from build123d import *

# Parameters (mm, degrees)
SKETCH1_R                = 55.5
BOSS_EXTRUDE1_DEPTH      = 7
CUT_EXTRUDE1_DEPTH       = 7
FILLET1_R                = 5
CIRPATTERN1_COUNT        = 7
FILLET1_OF_CIRPATTERN1_R = 5
SKETCH3_R                = 5
BOSS_EXTRUDE2_DEPTH      = 4.1


with BuildPart() as part:
    # Sketch1 → Boss-Extrude1 (new body)
    with BuildSketch(Plane(origin=(0, 0, 0), x_dir=(1, 0, 0), z_dir=(0, 1, 0))):
        with Locations(Location((0, 0, 0), (0, 0, 270))):
            Circle(SKETCH1_R)
    extrude(amount=BOSS_EXTRUDE1_DEPTH)

    # Sketch2 → Cut-Extrude1 (cut)
    with BuildSketch(Plane(origin=(0, 7, 0), x_dir=(1, 0, 0), z_dir=(0, 1, 0))):
        with BuildLine():
            Line((0, 15), (0, 45.5))
            ThreePointArc((0, 45.5), (15.561916521, 42.756014246), (29.246836241, 34.855022162))
            Line((29.246836241, 34.855022162), (9.641814145, 11.490666647))
            ThreePointArc((9.641814145, 11.490666647), (5.13030215, 14.095389312), (0, 15))
        make_face()
    cut_extrude1 = extrude(amount=-CUT_EXTRUDE1_DEPTH, mode=Mode.SUBTRACT)

    # Fillet1
    fillet1_edges = [part.edges().sort_by_distance(p)[0] for p in [
        (9.641814145, 3.5, -11.490666647),
        (0, 3.5, -15),
        (0, 3.5, -45.5),
        (29.246836241, 3.5, -34.855022162),
    ]]
    fillet(fillet1_edges, radius=FILLET1_R)

    # CirPattern1: Cut-Extrude1 ×7 about axis
    cirpattern1_axis = Axis((0, 0, 0), (0, 1, 0))
    for i in range(1, CIRPATTERN1_COUNT):
        add(cut_extrude1.rotate(cirpattern1_axis, i * 360 / CIRPATTERN1_COUNT), mode=Mode.SUBTRACT)

    # Fillet1 of CirPattern1
    fillet1_of_cirpattern1_edges = [part.edges().sort_by_distance(p)[0] for p in [
        (-2.972192148, 3.5, -14.702587318),
        (-11.727472237, 3.5, -9.352347028),
        (-35.573332452, 3.5, -28.368785985),
        (-9.015649516, 3.5, -44.597848197),
        (-13.348077132, 3.5, -6.84315986),
        (-14.623918683, 3.5, 3.337814009),
        (-44.359220004, 3.5, 10.124702495),
        (-40.489167301, 3.5, -20.75758491),
        (-13.672587785, 3.5, 6.169306547),
        (-6.508256087, 3.5, 13.514533019),
        (-19.74171013, 3.5, 40.99408349),
        (-41.47351628, 3.5, 18.713563192),
        (-3.701360965, 3.5, 14.536159293),
        (6.508256087, 3.5, 13.514533019),
        (19.74171013, 3.5, 40.99408349),
        (-11.227461595, 3.5, 44.093016523),
        (9.057066155, 3.5, 11.956987608),
        (14.623918683, 3.5, 3.337814009),
        (44.359220004, 3.5, 10.124702495),
        (27.47310067, 3.5, 36.269529079),
        (14.99533773, 3.5, 0.373960376),
        (11.727472237, 3.5, -9.352347028),
        (35.573332452, 3.5, -28.368785985),
        (45.485857781, 3.5, 1.134346474),
    ]]
    fillet(fillet1_of_cirpattern1_edges, radius=FILLET1_OF_CIRPATTERN1_R)

    # Sketch3 → Boss-Extrude2 (add)
    with BuildSketch(Plane(origin=(0, 7, 0), x_dir=(1, 0, 0), z_dir=(0, 1, 0))):
        with Locations(Location((0, 0, 0), (0, 0, 270))):
            Circle(SKETCH3_R)
    extrude(amount=BOSS_EXTRUDE2_DEPTH)


solid = part.part
Input: part model. Units: mm. Frame: model coordinates. Coordinates: 2 decimals unless noted, no trailing zeros. Loops run counter-clockwise (first coordinate to the right, second up) from the corner with the lowest first, then second, coordinate; pieces in that order, holes last. Notation, with made-up numbers: (-30.75, -8.5) -> (-15.75, -8.5) arc R24 cw to (-15.75, 18.5) -> close; hole circle Ø10 at (66.5, -11). An arc over 180 degrees is marked (long way). Write each question's results on one line, items separated by ' | '. Start each with the question number.
Q1. Ray query, line 1 (X direction, y = 0.5, z = -26.5); line 2 (Z direction, x = 35, y = 0.5); line 3 (X direction, y = 3.5, z = -37). Return the intervals inside material, ascending. Write a range as from..to.
Q2. Section D-D, the plane y = 2.5. State how many separate pieces and enclosed holes the cut face has, plus the area to 3 significant figures.
Q3. Section C-C, the plane y = 9. Return the cut outline in (x, z).
Q4. Section A-A, the plane z = 2.5. Return the cut outline in (x, y).
Q5. Pin query (flat end, axial travel): pin 1 (1 mm diameter, centred on y = 1.5, z = 8, fed in from -X); pin 2 (1 mm diameter, centred on y = 6.5, z = -35, fed in from +X); pin 3 (6 mm diameter, centred on x = 38.5, y = 6, fed in from +Z). Return the tip coordinate at first contact, or that it passes through.
Q6. Section B-B, the plane x = 22. Return the cut outline in (y, z), plus the area to 3 significant figures.
Found:
1) line 1: -48.76..-32.65, -5.36..0, 22.24..48.76 | line 2: -43.07..-26.13, 0.87..7.99, 29.07..43.07 | line 3: -41.37..-26.48, -7.48..0, 26..41.37
2) separate pieces: 1 | enclosed holes: 7 | area: 5,310 mm2
3) outline: circle Ø10 at (0, 0)
4) outline: (-55.44, 0) -> (-45.43, 0) -> (-45.43, 7) -> (-55.44, 7) -> close; (-16.04, 0) -> (55.44, 0) -> (55.44, 7) -> (4.33, 7) -> (4.33, 11.1) -> (-4.33, 11.1) -> (-4.33, 7) -> (-16.04, 7) -> close
5) pin 1: x = -54.99 | pin 2: x = 43.47 | pin 3: z = 42.66
6) outline: (0, -50.95) -> (7, -50.95) -> (7, -39.83) -> (0, -39.83) -> close; (0, -26.22) -> (7, -26.22) -> (7, -17.54) -> (0, -17.54) -> close; (0, 0.55) -> (7, 0.55) -> (7, 5.02) -> (0, 5.02) -> close; (0, 29.04) -> (7, 29.04) -> (7, 50.95) -> (0, 50.95) -> close | area: 323 mm2
